Verification items for the finished model (mm, model axes). A direction names the side the tool comes from. Round coordinates to 2 decimals unless told otherwise and drop trailing zeros. Order: outer loops, then holes, each group sorted by start corner. A loop starts at its lowest first (then second) coordinate and runs counter-clockwise, first axis right, second up. Notation, with made-up numbers: (-15, -9) -> (9, -9) arc R24 cw to (9, 21) -> close; hole circle Ø3 at (24.25, -0.5). An arc over 180 degrees is marked (long way). Put each result on its own line as item: value.
```python
from build123d import *

# Parameters (mm, degrees)
SKETCH1_W                = 17
SKETCH1_H                = 40
BOSS_EXTRUDE1_DEPTH      = 75
M4_CLEARANCE_HOLE1_D     = 4.5
M4_CLEARANCE_HOLE1_DEPTH = 15
M4_CLEARANCE_HOLE1_TIP   = 1.351936393
CUT_EXTRUDE1_DEPTH       = 3.3
M6_CLEARANCE_HOLE1_D     = 6.6
M6_CLEARANCE_HOLE1_DEPTH = 29
M6_CLEARANCE_HOLE1_TIP   = 1.982840043
CUT_EXTRUDE2_START       = -25
CUT_EXTRUDE2_DEPTH       = 5.5
SKETCH11_W               = 5.5
SKETCH11_H               = 10.2
CUT_EXTRUDE3_DEPTH       = 10
CHAMFER1_START           = -8.5
CHAMFER1_DEPTH           = 17
CHAMFER2_SIZE            = 2
CHAMFER3_SIZE            = 2


with BuildPart() as part:
    # Sketch1 → Boss-Extrude1 (new body)
    with BuildSketch(Plane.XY):
        Rectangle(SKETCH1_W, SKETCH1_H)
    extrude(amount=-BOSS_EXTRUDE1_DEPTH)

    # M4 Clearance Hole1
    with Locations(Plane(origin=(8.5, 0, 0), x_dir=(0, 0, -1), z_dir=(1, 0, 0))):
        with Locations((15, 8), (15, -8)):
            Hole(M4_CLEARANCE_HOLE1_D / 2, depth=M4_CLEARANCE_HOLE1_DEPTH)
            with Locations((0, 0, -(M4_CLEARANCE_HOLE1_DEPTH + M4_CLEARANCE_HOLE1_TIP / 2))):  # 118° drill point
                Cone(0, M4_CLEARANCE_HOLE1_D / 2, M4_CLEARANCE_HOLE1_TIP, mode=Mode.SUBTRACT)

    # Sketch6 → Cut-Extrude1 (cut)
    with BuildSketch(Plane.ZY.offset(8.5)):
        Polygon((-10.843078062, 8), (-12.921539031, 11.6), (-17.078460969, 11.6), (-19.156921938, 8), (-17.078460969, 4.4), (-12.921539031, 4.4), align=None)
        Polygon((-10.843078062, -8), (-12.921539031, -4.4), (-17.078460969, -4.4), (-19.156921938, -8), (-17.078460969, -11.6), (-12.921539031, -11.6), align=None)
    extrude(amount=-CUT_EXTRUDE1_DEPTH, mode=Mode.SUBTRACT)

    # M6 Clearance Hole1
    with Locations(Plane(origin=(0, 0, -75), x_dir=(-1, 0, 0), z_dir=(0, 0, -1))):
        with Locations((1.5, -10), (1.5, 10)):
            Hole(M6_CLEARANCE_HOLE1_D / 2, depth=M6_CLEARANCE_HOLE1_DEPTH)
            with Locations((0, 0, -(M6_CLEARANCE_HOLE1_DEPTH + M6_CLEARANCE_HOLE1_TIP / 2))):  # 118° drill point
                Cone(0, M6_CLEARANCE_HOLE1_D / 2, M6_CLEARANCE_HOLE1_TIP, mode=Mode.SUBTRACT)

    # Sketch10 → Cut-Extrude2 (cut)
    with BuildSketch(Plane(origin=(0, 0, -75), x_dir=(-1, 0, 0), z_dir=(0, 0, -1)).offset(CUT_EXTRUDE2_START)):
        Polygon((7.388972746, 10), (4.444486373, 15.1), (-1.444486373, 15.1), (-4.388972746, 10), (-1.444486373, 4.9), (4.444486373, 4.9), align=None)
        Polygon((7.388972746, -10), (4.444486373, -4.9), (-1.444486373, -4.9), (-4.388972746, -10), (-1.444486373, -15.1), (4.444486373, -15.1), align=None)
    extrude(amount=CUT_EXTRUDE2_DEPTH, mode=Mode.SUBTRACT)

    # Sketch11 → Cut-Extrude3 (cut)
    with BuildSketch(Plane(origin=(8.5, 0, 0), x_dir=(0, 0, -1), z_dir=(1, 0, 0))):
        with Locations((52.75, 10)):
            Rectangle(SKETCH11_W, SKETCH11_H)
        with Locations((52.75, -10)):
            Rectangle(SKETCH11_W, SKETCH11_H)
    extrude(amount=-CUT_EXTRUDE3_DEPTH, mode=Mode.SUBTRACT)

    # Chamfer1: read off the stored shape, not the designer's step
    # Chamfer1 outline → Chamfer1 (cut)
    with BuildSketch(Plane.YZ.offset(CHAMFER1_START)):
        Polygon((-5, -24.156921938), (-10, -29.156921938), (-10, -40), (-5, -45), (5, -45), (10, -40), (10, -29.156921938), (5, -24.156921938), align=None)
    extrude(amount=CHAMFER1_DEPTH, mode=Mode.SUBTRACT)

    # Chamfer2
    chamfer2_edges = [part.edges().sort_by_distance(p)[0] for p in [
        (-8.5, 20, -37.5),
        (8.5, 20, -37.5),
        (8.5, -20, -37.5),
        (-8.5, -20, -37.5),
    ]]
    chamfer(chamfer2_edges, length=CHAMFER2_SIZE)

    # Chamfer3
    chamfer3_edges = [part.edges().sort_by_distance(p)[0] for p in [
        (-8.5, -10, -34.578460969),
        (8.5, -10, -34.578460969),
        (-8.5, 0, -24.156921938),
        (8.5, 0, -24.156921938),
        (-8.5, 10, -34.578460969),
        (8.5, 10, -34.578460969),
        (-8.5, 0, -45),
        (8.5, 0, -45),
        (8.5, -7.5, -26.656921938),
        (-8.5, -7.5, -26.656921938),
        (8.5, 7.5, -26.656921938),
        (-8.5, 7.5, -26.656921938),
        (8.5, 7.5, -42.5),
        (-8.5, 7.5, -42.5),
        (8.5, -7.5, -42.5),
        (-8.5, -7.5, -42.5),
    ]]
    chamfer(chamfer3_edges, length=CHAMFER3_SIZE)


solid = part.part
```
Item 1: Depth check by flat-ended pin: pin 1 Ø3.5 at (y, z) = (-7, -13.5) entering from -X. Enter the tip coordinate at first touch or a pass-through.
Geometry check:
pin 1: x = -5.2
Item 2: Release check for a two-part mould opening along Z. For faces 6 (the face through (0, -20, -37)), 7 (the face through (-7.49, 8.24, -26)), 8 (the face through (0, 0, -75)) record: pulls with the +Z half, pulls with the -Z half, needs draft (parallel to the pull), parting line crosses it, or undercut.
Geometry check:
face 6: needs draft
face 7: undercut
face 8: pulls with the -Z half
Item 3: Sectioned sample at C-C, the plane y = 1.5. Record the boundary of the cut face in (x, z), then the cut area to 3 significant figures.
Geometry check:
outline: (-8.5, -75) -> (8.5, -75) -> (8.5, -47) -> (6.5, -45) -> (-6.5, -45) -> (-8.5, -47) -> close; (-8.5, -22.16) -> (-6.5, -24.16) -> (6.5, -24.16) -> (8.5, -22.16) -> (8.5, 0) -> (-8.5, 0) -> close
area: 913 mm2
Item 4: Sectioned sample at A-A, the plane z = -31. Record the boundary of the cut face in (x, y).
Geometry check:
outline: (-8.5, -18) -> (-6.5, -20) -> (6.5, -20) -> (8.5, -18) -> (8.5, -12) -> (6.5, -10) -> (-6.5, -10) -> (-8.5, -12) -> close; (-8.5, 12) -> (-6.5, 10) -> (6.5, 10) -> (8.5, 12) -> (8.5, 18) -> (6.5, 20) -> (-6.5, 20) -> (-8.5, 18) -> close
Item 5: Material ranges on line 1 along Y through (x, z) = (1, -53.5); line 2 along Y through (x, z) = (-1.5, -49.15); line 3 along Z through (x, y) = (-3.5, 5), recorded low to high.
Geometry check:
line 1: -20 to -15.1, -4.9 to 4.9, 15.1 to 20
line 2: -20 to -13.3, -6.7 to 6.7, 13.3 to 20
line 3: -75 to -55.5, -50 to -45, -24.16 to 0
Item 6: Sectioned sample at B-B, the plane z = -60. Record the boundary of the cut face in (x, y), then the cut area to 3 significant figures.
Geometry check:
outline: (-8.5, -18) -> (-6.5, -20) -> (6.5, -20) -> (8.5, -18) -> (8.5, 18) -> (6.5, 20) -> (-6.5, 20) -> (-8.5, 18) -> close; hole circle Ø6.6 at (-1.5, -10); hole circle Ø6.6 at (-1.5, 10)
area: 604 mm2
Item 7: Tool access check on faces 1 (the face through (-7.5, 19, -37)), 2 (the face through (1.55, -11.26, -65.11)), 3 (the face through (0, 0, -24.157)), 4 (the face through (-5.94, -7.49, -52.71)), 5 (the face through (-7, 11.6, -15)). Record the directions out of +Z, -Z, +X, -X, +Y, -Y that give a thin tool (end or side, any length) a straight path to the whole face; none if there is none.
Geometry check:
face 1: +Z, -Z, -X, +Y
face 2: -Z
face 3: +X, -X
face 4: +X
face 5: -X
